from build123d import *

# Parameters (mm, degrees)
SKETCH1_W            = 38.1
SKETCH1_H            = 38.1
BOSS_EXTRUDE1_DEPTH  = 6.35
SKETCH5_R            = 8
CUT_EXTRUDE1_DEPTH   = 55.254423783
M3_CLEARANCE_HOLE1_D = 3.4
SKETCH6_R            = 1.5875
CUT_EXTRUDE2_DEPTH   = 55.254423783
FILLET1_R            = 1.5875


with BuildPart() as part:
    # Sketch1 → Boss-Extrude1 (new body)
    with BuildSketch(Plane(origin=(0, 0, 0), x_dir=(1, 0, 0), z_dir=(0, 1, 0))):
        with Locations((-19.05, -19.05)):
            Rectangle(SKETCH1_W, SKETCH1_H)
    extrude(amount=BOSS_EXTRUDE1_DEPTH)

    # Sketch5 → Cut-Extrude1 (cut, through all)
    with BuildSketch(Plane(origin=(0, 6.35, 0), x_dir=(1, 0, 0), z_dir=(0, 1, 0))):
        with Locations(Location((-19.05, -19.05, 0), (0, 0, 270))):
            Circle(SKETCH5_R)
    extrude(amount=-CUT_EXTRUDE1_DEPTH, mode=Mode.SUBTRACT)

    # M3 Clearance Hole1 (through all)
    with Locations(Plane(origin=(0, 6.35, 0), x_dir=(-1, 0, 0), z_dir=(0, 1, 0))):
        with Locations((30.05074, 19.05), (24.55037, 9.5230797), (13.54963, 9.5230797), (8.04926, 19.05), (13.54963, 28.5769203), (24.55037, 28.5769203)):
            Hole(M3_CLEARANCE_HOLE1_D / 2)

    # Sketch6 → Cut-Extrude2 (cut, through all)
    with BuildSketch(Plane(origin=(0, 6.35, 0), x_dir=(1, 0, 0), z_dir=(0, 1, 0))):
        with Locations(Location((-34.925, -3.175, 0), (0, 0, 270))):
            Circle(SKETCH6_R)
        with Locations(Location((-3.175, -3.175, 0), (0, 0, 90))):
            Circle(SKETCH6_R)
        with Locations(Location((-3.175, -34.925, 0), (0, 0, 270))):
            Circle(SKETCH6_R)
        with Locations(Location((-34.925, -34.925, 0), (0, 0, 90))):
            Circle(SKETCH6_R)
    extrude(amount=-CUT_EXTRUDE2_DEPTH, mode=Mode.SUBTRACT)

    # Fillet1
    fillet1_edges = [part.edges().sort_by_distance(p)[0] for p in [
        (0, 3.175, 38.1),
        (-38.1, 3.175, 38.1),
        (-38.1, 3.175, 0),
        (0, 3.175, 0),
    ]]
    fillet(fillet1_edges, radius=FILLET1_R)


solid = part.part
CAD build for the part. Positions are in the model's coordinates, mm. Coordinates: 2 decimals unless noted, no trailing zeros. Write each loop counter-clockwise with the first axis right and the second up, starting at its lowest first coordinate (ties: lowest second). Pieces come first, ordered by that corner, then holes. Notation, with made-up numbers: (17.5, 60.5) - (46.5, 60.5) arc R32 ccw to (46.5, 91.5) - close; hole circle Ø8 at (15, -13.75). An arc over 180 degrees is marked (long way). Use a Markdown table: item, result. Add a question column.
Item 1: Band-saw the part on C-C, the plane z = 10. Give the cut face in (x, y).
Item 2: Flat gauge pins, fed straight in: pin 1 (5 mm diameter, centred on x = -34.925, z = 3.175, fed in from +Y); pin 2 (2 mm diameter, centred on x = -24.55, z = 9.52, fed in from +Y). Where does each tip first touch, or does it go through?
Item 3: Band-saw the part on D-D, the plane y = 2.5. Give the number of separate pieces and of enclosed holes in the cut face, and give its area (3 significant figures).
Item 4: Mould opens along Z. For faces 1 (the face through (-0.48, 3.22, 37.65)), 2 (the face through (0, 3, 19)), 3 (the face through (-22.98, 3.13, 27.93)) say: pulls with the +Z half, pulls with the -Z half, needs draft (parallel to the pull), parting line crosses it, or undercut.
Item 5: Drill centre lines: L1, parallel to Z at x = -35, y = 2.75; L2, parallel to Z at x = -34, y = 1.5; L3, parallel to X at y = 3.75, z = 30. Where is each one in solid material? Low to high. Write a range as from..to.
Item 6: Band-saw the part on A-A, the plane z = 19.05. Give the cut face in (x, y), and give its area (3 significant figures).
Item 7: Band-saw the part on B-B, the plane x = -19.05. Give the cut face in (y, z), and give its area (3 significant figures).
Numbers:
| question | item | result |
|---|---|---|
| 1 | outline | (-38.1, 0) - (-26.18, 0) - (-26.18, 6.35) - (-38.1, 6.35) - close; (-22.92, 0) - (-15.18, 0) - (-15.18, 6.35) - (-22.92, 6.35) - close; (-11.92, 0) - (0, 0) - (0, 6.35) - (-11.92, 6.35) - close |
| 2 | pin 1 | y = 6.35 |
| 2 | pin 2 | through |
| 3 | separate pieces | 1 |
| 3 | enclosed holes | 11 |
| 3 | area | 1,160 mm2 |
| 4 | face 1 | pulls with the +Z half |
| 4 | face 2 | needs draft |
| 4 | face 3 | undercut |
| 5 | L1 | 0..1.59, 4.76..33.34, 36.51..38.1 |
| 5 | L2 | 0..1.88, 4.47..33.63, 36.22..38.1 |
| 5 | L3 | -38.1..-25.48, -23.62..-14.48, -12.62..0 |
| 6 | outline | (-38.1, 0) - (-31.75, 0) - (-31.75, 6.35) - (-38.1, 6.35) - close; (-28.35, 0) - (-27.05, 0) - (-27.05, 6.35) - (-28.35, 6.35) - close; (-11.05, 0) - (-9.75, 0) - (-9.75, 6.35) - (-11.05, 6.35) - close; (-6.35, 0) - (0, 0) - (0, 6.35) - (-6.35, 6.35) - close |
| 6 | area | 97.2 mm2 |
| 7 | outline | (0, 0) - (6.35, 0) - (6.35, 11.05) - (0, 11.05) - close; (0, 27.05) - (6.35, 27.05) - (6.35, 38.1) - (0, 38.1) - close |
| 7 | area | 140 mm2 |
